```python
from build123d import *

# Parameters (mm, degrees)
MAIN_BODY_DEPTH             = 15
M5_HOLE_REACH               = 145.788
SKETCH2_R                   = 2.725
GRIP_REACH                  = 134.853
SKETCH8_W                   = 7.2
SKETCH8_H                   = 7.2
BUTTON_1_DEPTH              = 7
SKETCH9_R                   = 2
HOLE_WIRES_BUTTON_1_DEPTH   = 3
OUTER_FILLET_R              = 10
SKETCH13_W                  = 7.2
SKETCH13_H                  = 7.2
BUTTON_2_DEPTH              = 10
BUTTONS_FILLET_R            = 1
SKETCH16_R                  = 2
WIRE_ROUTING_DEPTH          = 40
M5_NUT_DEPTH                = 6
SKETCH18_W                  = 15
SKETCH18_H                  = 3
DOVETAIL_MALE_SLOT_DEPTH    = 4
DOVETAIL_MALE_SLOT_FILLET_R = 2


with BuildPart() as part:
    # Model → Main Body (new body)
    with BuildSketch(Plane.XY):
        Polygon((80, 115), (80, 105), (10, 105), (10, 10), (80, 10), (80, 0), (0, 0), (0, 22.5), (-5, 22.5), (-5, 92.5), (0, 92.5), (0, 115), align=None)
    extrude(amount=MAIN_BODY_DEPTH)

    # Sketch2 → M5 Hole (cut, up to next)
    with BuildSketch(Plane.ZY.offset(5), mode=Mode.PRIVATE) as m5_hole_sk1:
        with Locations((7.5, 57.5)):
            Circle(SKETCH2_R)
    m5_hole_tool1 = extrude(m5_hole_sk1.sketch, amount=-M5_HOLE_REACH, mode=Mode.PRIVATE) & part.part
    add(m5_hole_tool1.solids().sort_by_distance((-5, 57.5, 7.5))[0], mode=Mode.SUBTRACT)

    # Sketch6 → Grip (add, up to next)
    with BuildSketch(Plane.XZ.offset(-105), mode=Mode.PRIVATE) as grip_sk1:
        with BuildLine():
            Line((52.009621164, 15), (77.990380713, 15))
            ThreePointArc((77.990380713, 15), (80, 7.5), (77.990380713, 0))
            Line((77.990380713, 0), (52.009621164, 0))
            ThreePointArc((52.009621164, 0), (50.000002221, 7.5), (52.009621164, 15))
        make_face()
    grip_tool1 = extrude(grip_sk1.sketch, amount=GRIP_REACH, mode=Mode.PRIVATE) - part.part
    add(grip_tool1.solids().sort_by_distance((65.000001, 105, 7.5))[0])

    # Sketch8 → Button 1 (cut)
    with BuildSketch(Plane(origin=(0, 115, 0), x_dir=(1, 0, 0), z_dir=(0, 1, 0))):
        with Locations((49.9, -7.6)):
            Rectangle(SKETCH8_W, SKETCH8_H)
    extrude(amount=-BUTTON_1_DEPTH, mode=Mode.SUBTRACT)

    # Sketch9 → Hole Wires Button 1 (cut)
    with BuildSketch(Plane(origin=(0, 108, 0), x_dir=(1, 0, 0), z_dir=(0, 1, 0))):
        with Locations(Location((49.798571137, -7.7, 0), (0, 0, 270))):
            Circle(SKETCH9_R)
    extrude(amount=-HOLE_WIRES_BUTTON_1_DEPTH, mode=Mode.SUBTRACT)

    # Outer Fillet
    # the kernel refuses this fillet: 10 mm, written as the material it adds along each edge
    with BuildSketch(Plane(origin=(0, 22.5, 0), x_dir=(-1, 0, 0), z_dir=(0, 0, 1))) as outer_fillet_piece_1:
        with BuildLine():
            CenterArc((10, 8.660254038), OUTER_FILLET_R, 180, 60)
            Line((0, 8.660254038), (0, 0))
            Line((0, 0), (5, 0))
        make_face()
    extrude(amount=15)
    with BuildSketch(Plane(origin=(10, 10, 0), x_dir=(1, 0, 0), z_dir=(0, 0, 1)), Plane(origin=(10, 105, 0), x_dir=(0, -1, 0), z_dir=(0, 0, 1))) as outer_fillet_piece_2:
        with BuildLine():
            CenterArc((OUTER_FILLET_R, OUTER_FILLET_R), OUTER_FILLET_R, 180, 90)
            Line((0, OUTER_FILLET_R), (0, 0))
            Line((0, 0), (OUTER_FILLET_R, 0))
        make_face()
    extrude(amount=15)
    with BuildSketch(Plane(origin=(0, 92.5, 0), x_dir=(0, 1, 0), z_dir=(0, 0, 1))) as outer_fillet_piece_3:
        with BuildLine():
            CenterArc((8.660254038, 10), OUTER_FILLET_R, 210, 60)
            Line((0, 5), (0, 0))
            Line((0, 0), (8.660254038, 0))
        make_face()
    extrude(amount=15)
    # the kernel refuses this fillet: 10 mm, written as the material it takes off along each edge
    with BuildSketch(Plane(origin=(80, 115, -25), x_dir=(0, -1, 0), z_dir=(0, 0, 1)), Plane(origin=(80, 0, -25), x_dir=(-1, 0, 0), z_dir=(0, 0, 1)), Plane(origin=(0, 0, -25), x_dir=(0, 1, 0), z_dir=(0, 0, 1)), Plane(origin=(0, 115, -25), x_dir=(1, 0, 0), z_dir=(0, 0, 1))) as outer_fillet_2_piece_1:
        with BuildLine():
            CenterArc((OUTER_FILLET_R, -OUTER_FILLET_R), OUTER_FILLET_R, 90, 90)
            Line((0, -OUTER_FILLET_R), (0, 0))
            Line((0, 0), (OUTER_FILLET_R, 0))
        make_face()
    extrude(amount=65, mode=Mode.SUBTRACT)

    # Sketch13 → Button 2 (cut)
    with BuildSketch(Plane(origin=(0, 0, 0), x_dir=(-1, 0, 0), z_dir=(0, 0, -1))):
        with Locations((-10.1, 108.4)):
            Rectangle(SKETCH13_W, SKETCH13_H)
    extrude(amount=-BUTTON_2_DEPTH, mode=Mode.SUBTRACT)

    # Buttons Fillet
    buttons_fillet_edges = [part.edges().sort_by_distance(p)[0] for p in [
        (6.5, 112, 5),
        (6.5, 104.8, 5),
        (13.7, 104.8, 5),
        (13.7, 112, 5),
        (53.5, 111.5, 4),
        (53.5, 111.5, 11.2),
        (46.3, 111.5, 11.2),
        (46.3, 111.5, 4),
    ]]
    fillet(buttons_fillet_edges, radius=BUTTONS_FILLET_R)

    # Sketch16 → Wire Routing (cut, symmetric)
    with BuildSketch(Plane(origin=(10, 0, 0), x_dir=(0, 0, -1), z_dir=(1, 0, 0))):
        with Locations((-7.5, 105)):
            Circle(SKETCH16_R)
    extrude(amount=WIRE_ROUTING_DEPTH, both=True, mode=Mode.SUBTRACT)

    # Sketch17 → M5 Nut (cut)
    with BuildSketch(Plane(origin=(10, 0, 0), x_dir=(0, 0, -1), z_dir=(1, 0, 0))):
        Polygon((-7.5, 62.234272207), (-11.6, 59.867136104), (-11.6, 55.132863896), (-7.5, 52.765727793), (-3.4, 55.132863896), (-3.4, 59.867136104), align=None)
    extrude(amount=-M5_NUT_DEPTH, mode=Mode.SUBTRACT)

    # Sketch18 → Dovetail Male Slot (add)
    with BuildSketch(Plane.ZY.offset(5)):
        with Locations((7.5, 78.2)):
            Rectangle(SKETCH18_W, SKETCH18_H)
        with Locations((7.5, 36.8)):
            Rectangle(SKETCH18_W, SKETCH18_H)
    extrude(amount=DOVETAIL_MALE_SLOT_DEPTH)

    # Dovetail Male Slot Fillet
    dovetail_male_slot_fillet_edges = [part.edges().sort_by_distance(p)[0] for p in [
        (-5, 79.7, 7.5),
        (-5, 35.3, 7.5),
    ]]
    fillet(dovetail_male_slot_fillet_edges, radius=DOVETAIL_MALE_SLOT_FILLET_R)


solid = part.part
```
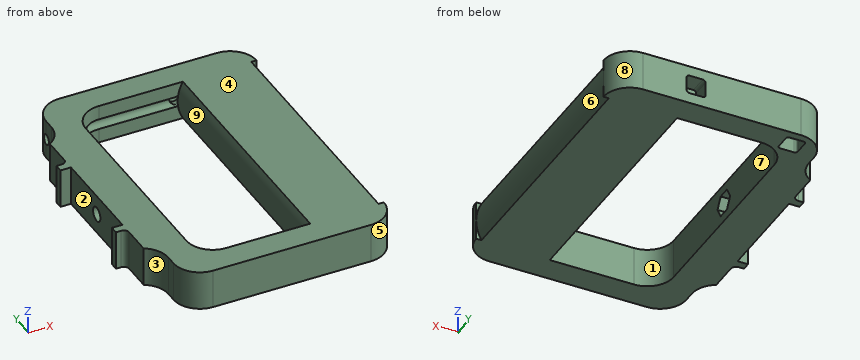
CAD build for the part. Positions are in the model's coordinates, mm. Face numbers are marked on the shaded views. A direction names the side the tool comes from. Round coordinates to 2 decimals unless told otherwise and drop trailing zeros. Loops run counter-clockwise (first coordinate to the right, second up) from the corner with the lowest first, then second, coordinate; pieces in that order, holes last. Notation, with made-up numbers: (-29, 11.5) - (-2, 11.5) arc R15 cw to (-2, 18.5) - close; hole circle Ø6 at (28, -36). An arc over 180 degrees is marked (long way). Return JSON: item names as keys, results as strings. Group by question number.
Q1. Drill centre lines: line 1 along Y through (x, z) = (25, 7.5); line 2 along X through (y, z) = (45.5, 7.25); line 3 along Y through (x, z) = (17.5, 9.25). Where is each one in solid material? Low to high. Write a range as [from, to].
Q2. Two-plate mould, pull along Y, no slides. Class the marked faces 1, 2, 3 and 4: +Y half, -Y half, draft (parallel to the pull), parting line (faces both ways), or undercut.
Q3. Tool access for the marked faces 5, 6, 7, 8 and 9: list every direction of +Z, -Z, +X, -X, +Y, -Y with a clear straight run to the whole face (end or side of a thin tool).
Q4. Band-saw the part on A-A on y = 12. Give the cut face in (x, z).
Q5. Band-saw the part on C-C on x = 28. Give the cut face in (y, z), plus the area to 3 significant figures.
Q6. Flat gauge pins, fed straight in: pin 1 Ø5.5 at (y, z) = (110.5, 8.5) entering from +X; pin 2 Ø2 at (x, z) = (79.5, 2.5) entering from -Y; pin 3 Ø8.5 at (y, z) = (57.5, 7.5) entering from -X. Where does each tip first touch, or does it go through?
Q7. Band-saw the part on D-D on y = 27.5. Give the cut face in (x, z), plus the area to 3 significant figures.
Q8. Band-saw the part on B-B on y = 57.5. Give the cut face in (x, z) (3 decimals).
Solutions:
{
 "1": {"line 1": "y = [0, 10], [107, 115]", "line 2": "x = [-5, 10], [50, 80]", "line 3": "y = [0, 10.32], [105.97, 115]"},
 "2": {"face 1": "undercut", "face 2": "undercut", "face 3": "-Y half", "face 4": "draft"},
 "3": {"face 5": "+Z, -Z, +X, -Y", "face 6": "+X", "face 7": "+Z, -Z", "face 8": "+Z, -Z, +X, +Y", "face 9": "none"},
 "4": {"outline": "(0, 0) - (14, 0) - (14, 15) - (0, 15) - close; (52.01, 0) - (77.99, 0) arc R15 ccw to (77.99, 15) - (52.01, 15) arc R15 ccw to start"},
 "5": {"outline": "(0, 0) - (10, 0) - (10, 15) - (0, 15) - close; (105, 0) - (115, 0) - (115, 15) - (105, 15) - (105, 9.5) arc R2 cw to (105, 5.5) - close", "area": "294 mm^2"},
 "6": {"pin 1": "stops at x = 79.61", "pin 2": "stops at y = 4.73", "pin 3": "stops at x = -5"},
 "7": {"outline": "(-5, 0) - (10, 0) - (10, 15) - (-5, 15) - close; (52.01, 0) - (77.99, 0) arc R15 ccw to (77.99, 15) - (52.01, 15) arc R15 ccw to start", "area": "655 mm^2"},
 "8": {"outline": "(-5, 0) - (10, 0) - (10, 3.4) - (4, 3.4) - (4, 4.775) - (-5, 4.775) - close; (-5, 10.225) - (4, 10.225) - (4, 11.6) - (10, 11.6) - (10, 15) - (-5, 15) - close; (52.01, 0) - (77.99, 0) arc R15 ccw to (77.99, 15) - (52.01, 15) arc R15 ccw to start"}
}
